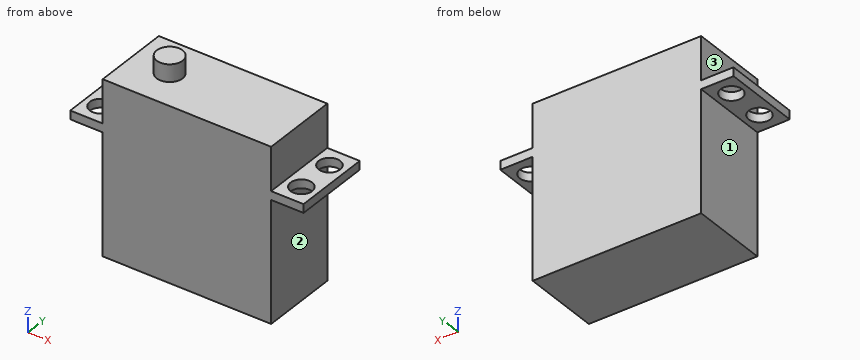
from build123d import *

# Parameters (mm, degrees)
SKETCH_1_W          = 54
SKETCH_1_H          = 18
EXTRUDE_1_DEPTH     = 2
SKETCH_2_W          = 39
SKETCH_2_H          = 18
EXTRUDE_2_DEPTH     = 10
SKETCH_3_R          = 3
EXTRUDE_3_DEPTH     = 4
SKETCH_4_W          = 39
SKETCH_4_H          = 18
EXTRUDE_4_DEPTH     = 28
SKETCH_6_R          = 2.5
CUT_EXTRUDE_1_DEPTH = 42.352146256


with BuildPart() as part:
    # 草图1 → 凸台-拉伸1 (new body)
    with BuildSketch(Plane.XY):
        Rectangle(SKETCH_1_W, SKETCH_1_H)
    extrude(amount=EXTRUDE_1_DEPTH)

    # 草图2 → 凸台-拉伸2 (add)
    with BuildSketch(Plane.XY.offset(2)):
        Rectangle(SKETCH_2_W, SKETCH_2_H)
    extrude(amount=EXTRUDE_2_DEPTH)

    # 草图3 → 凸台-拉伸3 (add)
    with BuildSketch(Plane.XY.offset(12)):
        with Locations((-10.5, 0)):
            Circle(SKETCH_3_R)
    extrude(amount=EXTRUDE_3_DEPTH)

    # 草图4 → 凸台-拉伸4 (add)
    with BuildSketch(Plane(origin=(0, 0, 0), x_dir=(-1, 0, 0), z_dir=(0, 0, -1))):
        Rectangle(SKETCH_4_W, SKETCH_4_H)
    extrude(amount=EXTRUDE_4_DEPTH)

    # 草图6 → 切除-拉伸1 (cut, through all)
    with BuildSketch(Plane.XY.offset(2)):
        with Locations((23.25, 4.5)):
            Circle(SKETCH_6_R)
        with Locations(Location((23.25, -4.5, 0), (0, 0, 180))):
            Circle(SKETCH_6_R)
        with Locations((-23.25, -4.5)):
            Circle(SKETCH_6_R)
        with Locations(Location((-23.25, 4.5, 0), (0, 0, 180))):
            Circle(SKETCH_6_R)
    extrude(amount=-CUT_EXTRUDE_1_DEPTH, mode=Mode.SUBTRACT)


solid = part.part
Geometry: final body of the model. Coordinates: model frame, mm. Face numbers are marked on the shaded views. A direction names the side the tool comes from. Coordinates: 2 decimals unless noted, no trailing zeros. Order: outer loops, then holes, each group sorted by start corner. A loop starts at its lowest first (then second) coordinate and runs counter-clockwise, first axis right, second up.
1) Set-up query: the marked faces 1, 2 and 3. Return all of +Z, -Z, +X, -X, +Y, -Y with unobstructed straight access to the full face (end or side cutting, diameter ignored); none if empty.
Result sheet:
face 1: -Z, -X, +Y, -Y
face 2: -Z, +X, +Y, -Y
face 3: +Z, -X, +Y, -Y
2) Section A-A (y = -4.5). Return loops of the section in (x, z), then the cut area to 3 significant figures.
Result sheet:
outline: (-27, 0) - (-25.75, 0) - (-25.75, 2) - (-27, 2) - close; (-20.75, 0) - (-19.5, 0) - (-19.5, -28) - (19.5, -28) - (19.5, 0) - (20.75, 0) - (20.75, 2) - (19.5, 2) - (19.5, 12) - (-19.5, 12) - (-19.5, 2) - (-20.75, 2) - close; (25.75, 0) - (27, 0) - (27, 2) - (25.75, 2) - close
area: 1,570 mm2
3) Ray query, probe 1 along Y at (x, z) = (23.25, 1.2); probe 2 along Z at (x, y) = (20, 5.5); probe 3 along X at (y, z) = (-2, 11). Return the intervals inside material, ascending.
Result sheet:
probe 1: y = -9 to -7, -2 to 2, 7 to 9
probe 2: z = 0 to 2
probe 3: x = -19.5 to 19.5
4) Section D-D (x = -10.5). Return loops of the section in (y, z), then the cut area to 3 significant figures.
Result sheet:
outline: (-9, -28) - (9, -28) - (9, 12) - (3, 12) - (3, 16) - (-3, 16) - (-3, 12) - (-9, 12) - close
area: 744 mm2
5) Section B-B (x = -23.25). Return loops of the section in (y, z).
Result sheet:
outline: (-9, 0) - (-7, 0) - (-7, 2) - (-9, 2) - close; (-2, 0) - (2, 0) - (2, 2) - (-2, 2) - close; (7, 0) - (9, 0) - (9, 2) - (7, 2) - close
6) First-contact query: P1, Ø5, axis at x = -4.5, y = 7, coming from the +Z side; P2, Ø8, axis at y = -3.5, z = 9, coming from the +X side; P3, Ø6.5, axis at x = 23.25, y = 4.5, coming from the +Z side. Flat tips, straight axial feed; report the tip coordinate or a pass-through.
Result sheet:
P1: stops at z = 12
P2: stops at x = 19.5
P3: stops at z = 2
7) Section C-C (y = 0). Return loops of the section in (x, z), then the cut area to 3 significant figures.
Result sheet:
outline: (-27, 0) - (-19.5, 0) - (-19.5, -28) - (19.5, -28) - (19.5, 0) - (27, 0) - (27, 2) - (19.5, 2) - (19.5, 12) - (-7.5, 12) - (-7.5, 16) - (-13.5, 16) - (-13.5, 12) - (-19.5, 12) - (-19.5, 2) - (-27, 2) - close
area: 1,610 mm2
